Could you check a few things on this drawing? It's one solid part, dimensions in mm from its lowest x, y, z. Give positions to 0.01 mm unless a question says otherwise; leave off trailing zeros. Loops run counter-clockwise (first coordinate to the right, second up) from the corner with the lowest first, then second, coordinate; pieces in that order, holes last. Notation, with made-up numbers: M -20.75,-23 L 11.25,-23 A20 ccw 11.25,0 Z; hole C 60,21 d4. An arc over 180 degrees is marked long. Answer in a Markdown table with one row per item. Add a question column.
1. If we section it at C-C on y = 5.25: List the corners of the cut face in (x, z) for me.
2. Thinking about a two-plate mould opening in Y: for the marked faces 1, 2, 3 and 4, which applies, released by +Y, released by -Y, zero draft, split by the parting line, or undercut?
3. If we section it at D-D on y = 0.5: List the corners of the cut face in (x, z) for me.
4. I need wall thicknesses on line 1 along X through (y, z) = (2.75, 0.7); line 2 along Y through (x, z) = (3, 1.9); line 3 along X through (y, z) = (1.5, 1.2) (1 decimal). Which ranges of each line are inside material? Lowest first, please. Write a range as from..to.
5. I'm going to push a flat-ended pin straight in: pin 1 Ø1 at (y, z) = (2.5, 2.5) entering from +X (1 decimal). Where does the tip first touch, or does it pass through?
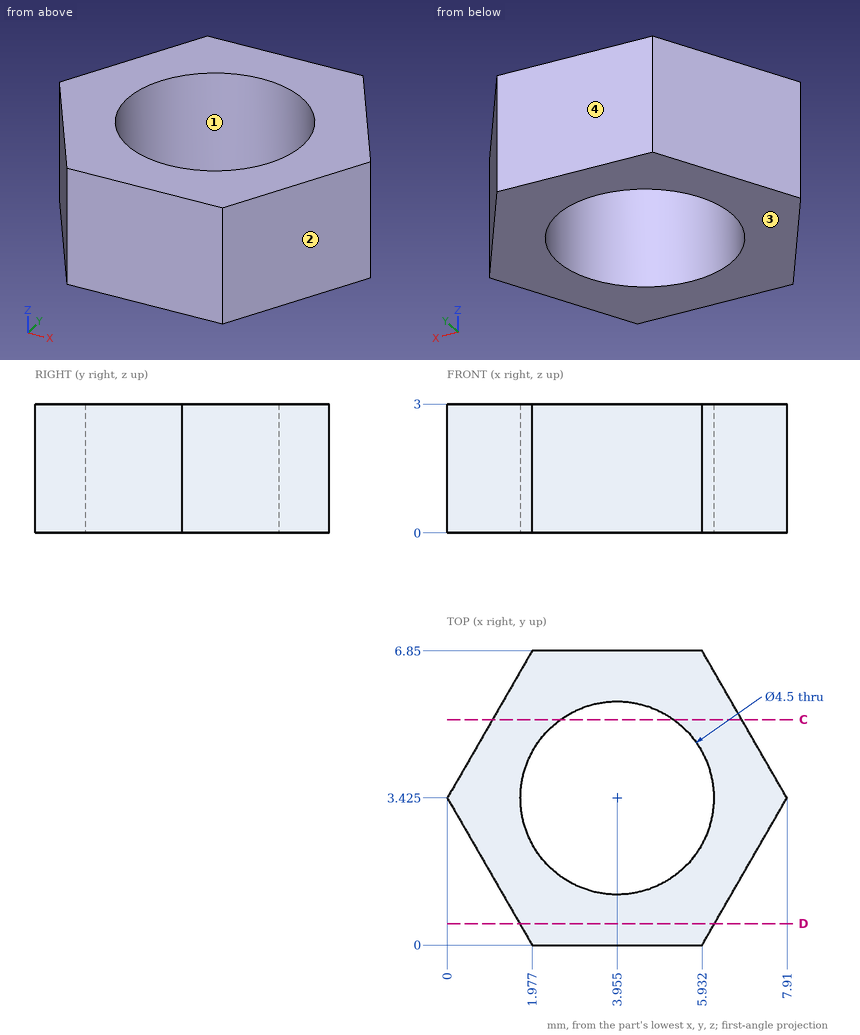
Results:
| question | item | result |
|---|---|---|
| 1 | outline | M 1.05,0 L 2.64,0 L 2.64,3 L 1.05,3 Z; M 5.27,0 L 6.86,0 L 6.86,3 L 5.27,3 Z |
| 2 | face 1 | undercut |
| 2 | face 2 | released by -Y |
| 2 | face 3 | zero draft |
| 2 | face 4 | released by +Y |
| 3 | outline | M 1.69,0 L 6.22,0 L 6.22,3 L 1.69,3 Z |
| 4 | line 1 | 0.39..1.81, 6.1..7.52 |
| 4 | line 2 | 0..1.39, 5.46..6.85 |
| 4 | line 3 | 1.1..2.8, 5.1..6.8 |
| 5 | pin 1 | x = 7.7 |
